Can you work these out from the model? Positions are in its coordinate system, mm. Face numbers are marked on the shaded views. Give positions to 0.01 mm unless a question says otherwise; leave off trailing zeros. Loops run counter-clockwise (first coordinate to the right, second up) from the corner with the lowest first, then second, coordinate; pieces in that order, holes last. Notation, with made-up numbers: M 71.25,-21.75 L 88.25,-21.75 A27 cw 88.25,-2.75 Z; hole C 74,0.5 d8. An arc over 180 degrees is marked long. Answer as a JSON object with one key per item and string values.
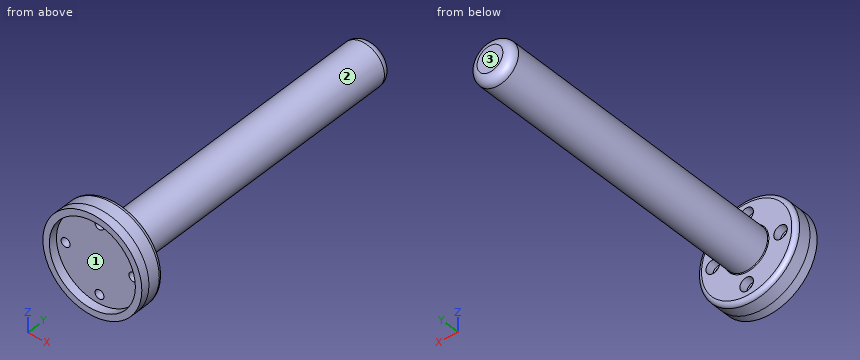
```python
from build123d import *

# Parameters (mm, degrees)
SKETCH1_R               = 36.5125
SKETCH1_R_2             = 31.75
BOSS_EXTRUDE1_DEPTH     = 6.35
SKETCH1_2_R             = 36.5125
BOSS_EXTRUDE2_DEPTH     = 12.35
SKETCH2_R               = 3.3
CUT_EXTRUDE1_DEPTH      = 1
CUT_EXTRUDE1_DEPTH_BACK = 19.7
SKETCH3_R               = 15.875
BOSS_EXTRUDE3_DEPTH     = 228.6
SKETCH4_R               = 5
CUT_EXTRUDE2_DEPTH      = 229.6
CUT_EXTRUDE2_DEPTH_BACK = 6
FILLET2_R               = 0.508
FILLET3_R               = 3.175
SKETCH5_R               = 9.525
CUT_EXTRUDE3_DEPTH      = 222.25
FILLET4_R               = 6.35
SKETCH6_R               = 15.875
BOSS_EXTRUDE4_DEPTH     = 6.35
FILLET5_R               = 6.35


with BuildPart() as part:
    # Sketch1 → Boss-Extrude1 (new body)
    with BuildSketch(Plane(origin=(0, 0, 0), x_dir=(1, 0, 0), z_dir=(0, 1, 0))):
        Circle(SKETCH1_R)
        Circle(SKETCH1_R_2, mode=Mode.SUBTRACT)
    extrude(amount=-BOSS_EXTRUDE1_DEPTH)

    # Sketch1<2> → Boss-Extrude2 (add)
    with BuildSketch(Plane(origin=(0, 0, 0), x_dir=(1, 0, 0), z_dir=(0, 1, 0))):
        Circle(SKETCH1_2_R)
    extrude(amount=BOSS_EXTRUDE2_DEPTH)

    # Sketch2 → Cut-Extrude1 (cut, two sides)
    with BuildSketch(Plane(origin=(0, 12.35, 0), x_dir=(1, 0, 0), z_dir=(0, 1, 0))) as cut_extrude1_sk:
        with Locations((0, 25)):
            Circle(SKETCH2_R)
        with Locations((25, 0)):
            Circle(SKETCH2_R)
        with Locations((0, -25)):
            Circle(SKETCH2_R)
        with Locations((-25, 0)):
            Circle(SKETCH2_R)
    extrude(amount=CUT_EXTRUDE1_DEPTH, mode=Mode.SUBTRACT)
    extrude(cut_extrude1_sk.sketch, amount=-CUT_EXTRUDE1_DEPTH_BACK, mode=Mode.SUBTRACT)

    # Sketch3 → Boss-Extrude3 (add)
    with BuildSketch(Plane(origin=(0, 12.35, 0), x_dir=(1, 0, 0), z_dir=(0, 1, 0))):
        Circle(SKETCH3_R)
    extrude(amount=BOSS_EXTRUDE3_DEPTH)

    # Sketch4 → Cut-Extrude2 (cut, two sides)
    with BuildSketch(Plane(origin=(0, 12.35, 0), x_dir=(1, 0, 0), z_dir=(0, 1, 0))) as cut_extrude2_sk:
        with Locations((-25, 0)):
            Circle(SKETCH4_R)
        with Locations((0, 25)):
            Circle(SKETCH4_R)
        with Locations((25, 0)):
            Circle(SKETCH4_R)
        with Locations((0, -25)):
            Circle(SKETCH4_R)
    extrude(amount=CUT_EXTRUDE2_DEPTH, mode=Mode.SUBTRACT)
    extrude(cut_extrude2_sk.sketch, amount=-CUT_EXTRUDE2_DEPTH_BACK, mode=Mode.SUBTRACT)

    # Fillet2
    fillet2_edges = [part.edges().sort_by_distance(p)[0] for p in [
        (-15.875, 12.35, 0),
    ]]
    fillet(fillet2_edges, radius=FILLET2_R)

    # Fillet3
    fillet3_edges = [part.edges().sort_by_distance(p)[0] for p in [
        (-36.5125, 12.35, 0),
    ]]
    fillet(fillet3_edges, radius=FILLET3_R)

    # Sketch5 → Cut-Extrude3 (cut)
    with BuildSketch(Plane(origin=(0, 240.95, 0), x_dir=(1, 0, 0), z_dir=(0, 1, 0))):
        Circle(SKETCH5_R)
    extrude(amount=-CUT_EXTRUDE3_DEPTH, mode=Mode.SUBTRACT)

    # Fillet4
    fillet4_edges = [part.edges().sort_by_distance(p)[0] for p in [
        (-9.525, 18.7, 0),
    ]]
    fillet(fillet4_edges, radius=FILLET4_R)

    # Sketch6 → Boss-Extrude4 (add)
    with BuildSketch(Plane(origin=(0, 240.95, 0), x_dir=(1, 0, 0), z_dir=(0, 1, 0))):
        Circle(SKETCH6_R)
    extrude(amount=-BOSS_EXTRUDE4_DEPTH)

    # Fillet5
    fillet5_edges = [part.edges().sort_by_distance(p)[0] for p in [
        (-15.875, 240.95, 0),
        (-9.525, 234.6, 0),
    ]]
    fillet(fillet5_edges, radius=FILLET5_R)


solid = part.part
```
1) Suppose I cut it at A-A, the plane x = 0. Give the number of separate pieces and of enclosed holes in the cut face, and give its area (3 significant figures).
Answer list:
{"separate pieces": "3", "enclosed holes": "1", "area": "3,920 mm^2"}
2) Please list where these lines run through material, in increasing order: line 1 along X through (y, z) = (1, 0); line 2 along Z through (x, y) = (0, 8); line 3 along Y through (x, z) = (1, -1). Write a range as from..to.
Answer list:
{"line 1": "-36.51..-28.3, -21.7..21.7, 28.3..36.51", "line 2": "-36.51..-30, -20..20, 30..36.51", "line 3": "0..18.7, 234.6..240.95"}
3) If we mould it in two halves opening along X, with no side actions, what happens to the marked faces 1, 2 and 3? For each: +X half, -X half, draft (parallel to the pull), parting line (faces both ways), or undercut.
Answer list:
{"face 1": "undercut", "face 2": "parting line", "face 3": "draft"}
4) Suppose I cut it at C-C, the plane y = 80. Write out the boundary of the cut face in (x, z) (3 decimals).
Answer list:
{"outline": "C 0,0 d31.75; hole C 0,0 d19.05"}
5) Will these pins go through, and if not, where does the flat tip stop? pin 1 Ø9 at (x, z) = (-25, 0) entering from -Y; pin 2 Ø10 at (y, z) = (59.5, -10) entering from -X; pin 3 Ø5 at (y, z) = (89.5, -8.5) entering from +X.
Answer list:
{"pin 1": "y = 0", "pin 2": "x = -15.07", "pin 3": "x = 14.7"}
